CAD build for the part. Positions are in the model's coordinates, mm. A direction names the side the tool comes from. Give positions to 0.01 mm unless a question says otherwise; leave off trailing zeros. Loops run counter-clockwise (first coordinate to the right, second up) from the corner with the lowest first, then second, coordinate; pieces in that order, holes last.
Item 1: Mould opens along X. For faces 1 (the flat face through (-5, 0, 15)), 2 (the cylindrical face through (-6.3, -1.2, 16.4)), 3 (the flat face through (0, 0, 11)), 4 (the flat face through (-7.5, 0, 11)) say: released by +X, released by -X, zero draft, split by the parting line, or undercut.
Item 2: Saw through at B-B on z = 18. Give the cut face in (x, y).
Item 3: Saw through at C-C on y = 0. Give the cut face in (x, z), plus the area to 3 significant figures.
Item 4: Saw through at D-D on x = -6. Give the cut face in (y, z).
Item 5: Which spindle directions (+Z, -Z, +X, -X, +Y, -Y) get a long thin tool onto all of the face, cutting with end or side? Do faces 5 (the flat face through (0, 7.5, 8)), 6 (the flat face through (5, 0, 15)). Say none if no direction does.
Item 6: Drop flat-ended pins along their axis: P1, Ø5, axis at x = -1.5, y = 5.5, coming from the +Z side; P2, Ø3.5, axis at y = 0, z = 18, coming from the -X side. Give the stop position or say it passes through.
Item 7: Probe probe 1 along X at (y, z) = (1.75, 15); probe 2 along Y at (x, z) = (-6.3, 18); probe 3 along Z at (x, y) = (-2.5, -1.25). List the from-to ranges inside material, lowest first.
Item 8: Saw through at A-A on z = 14. Give the cut face in (x, y), plus the area to 3 significant figures.
from build123d import *

# Parameters (mm, degrees)
SKETCH2_W           = 15
SKETCH2_H           = 15
BOSS_EXTRUDE2_DEPTH = 22
SKETCH4_W           = 10
SKETCH4_H           = 15
CUT_EXTRUDE1_DEPTH  = 11
SKETCH5_R           = 2
CUT_EXTRUDE2_DEPTH  = 25


with BuildPart() as part:
    # Sketch2 → Boss-Extrude2 (new body)
    with BuildSketch(Plane.XY):
        Rectangle(SKETCH2_W, SKETCH2_H)
    extrude(amount=BOSS_EXTRUDE2_DEPTH)

    # Sketch4 → Cut-Extrude1 (cut)
    with BuildSketch(Plane.XY.offset(22)):
        Rectangle(SKETCH4_W, SKETCH4_H)
    extrude(amount=-CUT_EXTRUDE1_DEPTH, mode=Mode.SUBTRACT)

    # Sketch5 → Cut-Extrude2 (cut)
    with BuildSketch(Plane.ZY.offset(7.5)):
        with Locations((18, 0)):
            Circle(SKETCH5_R)
    extrude(amount=-CUT_EXTRUDE2_DEPTH, mode=Mode.SUBTRACT)


solid = part.part
Results below:
1. face 1: undercut
1. face 2: zero draft
1. face 3: undercut
1. face 4: released by -X
2. outline: (-7.5, -7.5) - (-5, -7.5) - (-5, -2) - (-7.5, -2) - close; (-7.5, 2) - (-5, 2) - (-5, 7.5) - (-7.5, 7.5) - close; (5, -7.5) - (7.5, -7.5) - (7.5, -2) - (5, -2) - close; (5, 2) - (7.5, 2) - (7.5, 7.5) - (5, 7.5) - close
3. outline: (-7.5, 0) - (7.5, 0) - (7.5, 16) - (5, 16) - (5, 11) - (-5, 11) - (-5, 16) - (-7.5, 16) - close; (-7.5, 20) - (-5, 20) - (-5, 22) - (-7.5, 22) - close; (5, 20) - (7.5, 20) - (7.5, 22) - (5, 22) - close
3. area: 200 mm2
4. outline: (-7.5, 0) - (7.5, 0) - (7.5, 22) - (-7.5, 22) - close; hole circle Ø4 at (0, 18)
5. face 5: +Z, -Z, +X, -X, +Y
5. face 6: +Z, +Y, -Y
6. P1: stops at z = 11
6. P2: passes through
7. probe 1: x = -7.5 to -5, 5 to 7.5
7. probe 2: y = -7.5 to -2, 2 to 7.5
7. probe 3: z = 0 to 11
8. outline: (-7.5, -7.5) - (-5, -7.5) - (-5, 7.5) - (-7.5, 7.5) - close; (5, -7.5) - (7.5, -7.5) - (7.5, 7.5) - (5, 7.5) - close
8. area: 75.0 mm2
